Answer from the drawing. Dimensions are ordinates in mm from the lowest x, y and z of the part. A direction names the side the tool comes from. Give positions to 0.01 mm unless a question says otherwise; leave off trailing zeros. Loops run counter-clockwise (first coordinate to the right, second up) from the corner with the lowest first, then second, coordinate; pieces in that order, holes last. Notation, with made-up numbers: (-22, 43) - (16, 43) arc R33 ccw to (16, 72) - close; hole circle Ø5 at (-20, 48). An arc over 180 degrees is marked (long way). Put each result on its own line as item: value. Start each with the question number.
1. A cutting plane is placed at A-A, the plane z = 65. Determine the outline of the cut face in (x, y), plus the area to 3 significant figures.
2. Given pin 1 Ø2 at (x, y) = (3.5, 19) entering from +Z; pin 2 Ø3 at (y, z) = (12.5, 53) entering from +X; pin 3 Ø8 at (y, z) = (20, 12.5) entering from -X, each flat-ended and moving along its own axis, determine where each tip first touches the part or whether it passes through.
3. For the marked faces 1, 2 and 3, determine the directions among +Z, -Z, +X, -X, +Y, -Y from which every point of the face is accessible in a straight line to the end or side of a thin tool.
4. A cutting plane is placed at B-B, the plane y = 27. Determine the outline of the cut face in (x, z), plus the area to 3 significant figures.
5. A cutting plane is placed at C-C, the plane x = 18.5. Determine the outline of the cut face in (y, z), plus the area to 3 significant figures.
6. A cutting plane is placed at D-D, the plane z = 40.5. Determine the outline of the cut face in (x, y).
7. Consider L1, parallel to X at y = 31.5, z = 63.5; L2, parallel to X at y = 4, z = 71.5; L3, parallel to Y at x = 10.75, z = 61.75. Determine where each line is inside the solid, lowest interval first. Write a range as from..to.
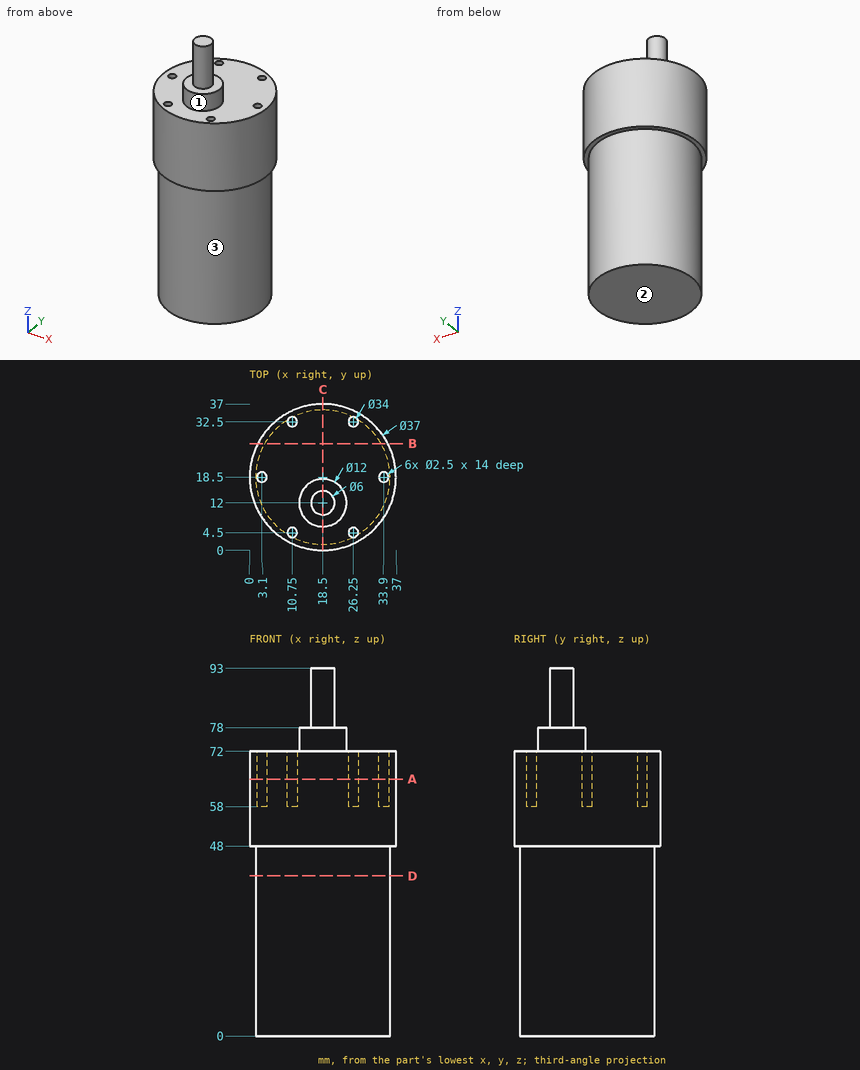
Return value:
1. outline: circle Ø37 at (18.5, 18.5); hole circle Ø2.5 at (3.1, 18.5); hole circle Ø2.5 at (10.75, 4.5); hole circle Ø2.5 at (10.75, 32.5); hole circle Ø2.5 at (26.25, 4.5); hole circle Ø2.5 at (26.25, 32.5); hole circle Ø2.5 at (33.9, 18.5)
1. area: 1,050 mm2
2. pin 1: stops at z = 72
2. pin 2: stops at x = 36.44
2. pin 3: stops at x = 1.5
3. face 1: +Z
3. face 2: -Z, +X, -X, +Y, -Y
3. face 3: -Z
4. outline: (2.07, 48) - (3.78, 48) - (3.78, 0) - (33.22, 0) - (33.22, 48) - (34.93, 48) - (34.93, 72) - (2.07, 72) - close
4. area: 2,200 mm2
5. outline: (0, 48) - (1.5, 48) - (1.5, 0) - (35.5, 0) - (35.5, 48) - (37, 48) - (37, 72) - (18, 72) - (18, 78) - (15, 78) - (15, 93) - (9, 93) - (9, 78) - (6, 78) - (6, 72) - (0, 72) - close
5. area: 2,680 mm2
6. outline: circle Ø34 at (18.5, 18.5)
7. L1: x = 5.34..10, 11.5..25.5, 27..31.66
7. L2: x = 7.01..9.6, 11.9..25.1, 27.4..29.99
7. L3: y = 1.7..3.25, 5.75..31.25, 33.75..35.3
